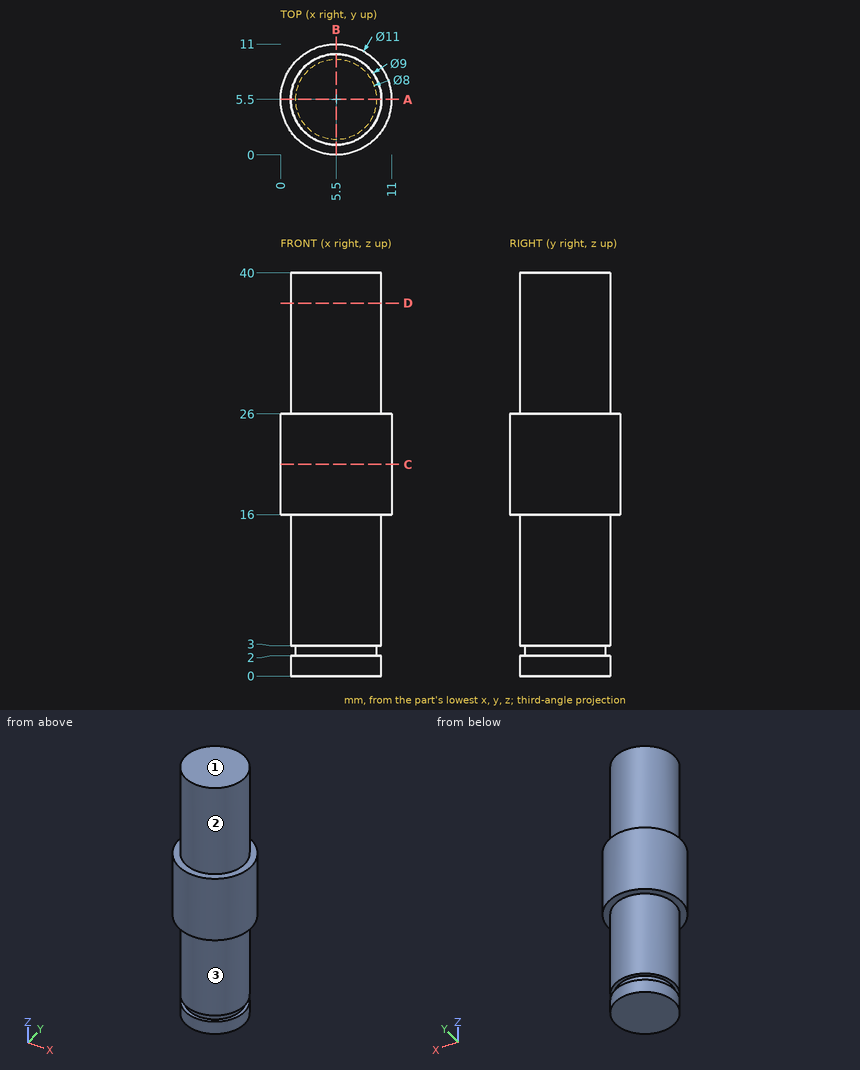
Verification items for this drawing (mm, ordinates from the low corner). A direction names the side the tool comes from. Round coordinates to 2 decimals unless told otherwise and drop trailing zeros. Write each loop counter-clockwise with the first axis right and the second up, starting at its lowest first coordinate (ties: lowest second). Pieces come first, ordered by that corner, then holes. Notation, with made-up numbers: (-3, 76.5) - (2, 76.5) arc R16 cw to (2, 91.5) - close; hole circle Ø11 at (4.5, 47). An arc over 180 degrees is marked (long way). One line per item, written item: value.
1. Cross-section at A-A on y = 5.5. Record the boundary of the cut face in (x, z).
The answers:
outline: (0, 16) - (1, 16) - (1, 3) - (1.5, 3) - (1.5, 2) - (1, 2) - (1, 0) - (10, 0) - (10, 2) - (9.5, 2) - (9.5, 3) - (10, 3) - (10, 16) - (11, 16) - (11, 26) - (10, 26) - (10, 40) - (1, 40) - (1, 26) - (0, 26) - close
2. Cross-section at C-C on z = 21. Record the boundary of the cut face in (x, y), and give its area (3 significant figures).
The answers:
outline: circle Ø11 at (5.5, 5.5)
area: 95.0 mm^2
3. Depth check by flat-ended pin: pin 1 Ø2 at (y, z) = (8, 22.5) entering from +X; pin 2 Ø3.5 at (x, y) = (5, 3.5) entering from -Z; pin 3 Ø3 at (y, z) = (7, 11) entering from +X; pin 4 Ø1.5 at (y, z) = (6.5, 9) entering from -X. Enter the tip coordinate at first touch or a pass-through.
The answers:
pin 1: stops at x = 10.79
pin 2: stops at z = 0
pin 3: stops at x = 10
pin 4: stops at x = 1.01
4. Set-up check for the marked faces 1, 2 and 3: record each of +Z, -Z, +X, -X, +Y, -Y from which the full face is reachable in a straight line by a thin tool's end or side.
The answers:
face 1: +Z, +X, -X, +Y, -Y
face 2: +Z
face 3: -Z
5. Scan lines: L1, parallel to Z at x = 1, y = 4.25; L2, parallel to Y at x = 5.5, z = 36.5; L3, parallel to X at y = 1.75, z = 20.5. Record each from-to range of solid material in increasing order.
The answers:
L1: z = 16 to 26
L2: y = 1 to 10
L3: x = 1.48 to 9.52
6. Cross-section at D-D on z = 37. Record the boundary of the cut face in (x, y), and give its area (3 significant figures).
The answers:
outline: circle Ø9 at (5.5, 5.5)
area: 63.6 mm^2
